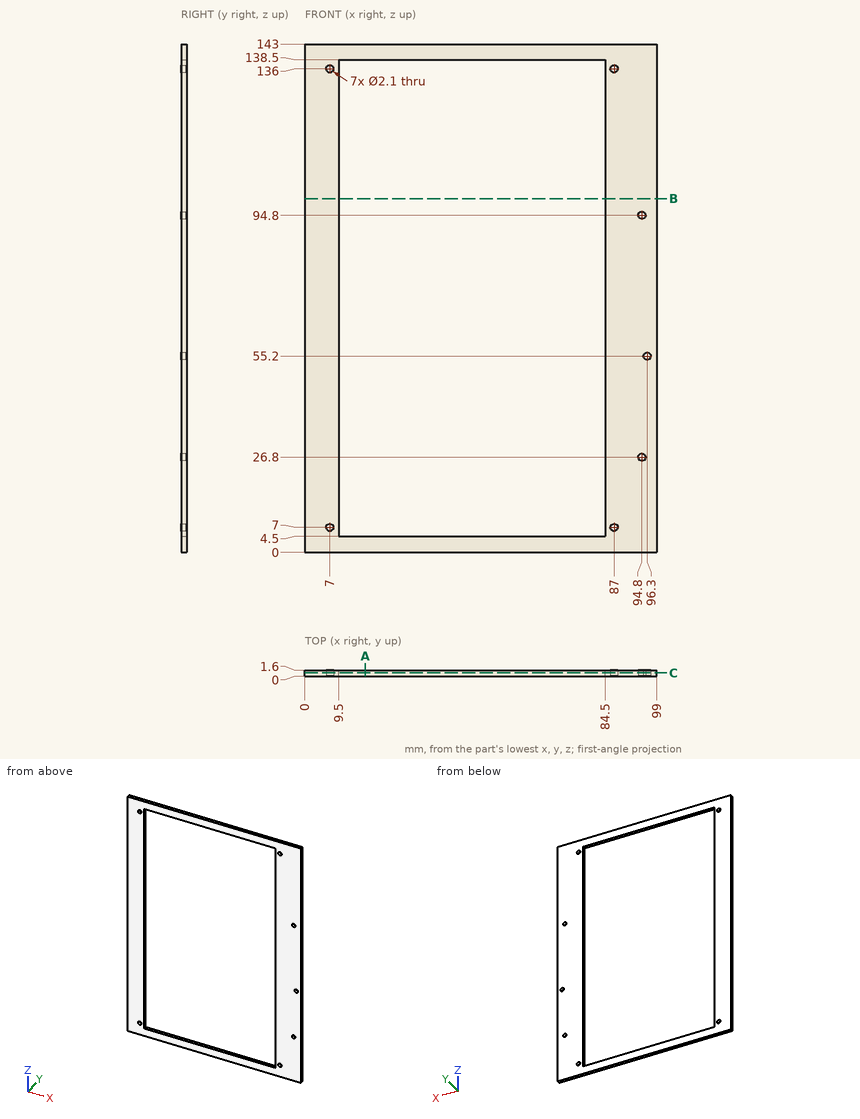
Drawing for the job (mm, zero at the part's lowest x, y, z). Coordinates: 2 decimals unless noted, no trailing zeros. Loops run counter-clockwise (first coordinate to the right, second up) from the corner with the lowest first, then second, coordinate; pieces in that order, holes last. Notation, with made-up numbers: (-39.5, -40) - (-13.5, -40) arc R31 cw to (-13.5, -3) - close; hole circle Ø8 at (-11, 20.25). An arc over 180 degrees is marked (long way). Use CSV: the item, a comma, the result in double quotes. Start each with the question number.
Q1. Drop a flat-ended pin along its axis: P1, Ø2.5, axis at x = 87, z = 7, coming from the +Y side. Give the stop position or say it passes through.
Q2. Cut at B-B, the plane z = 99.5. List the corners of the cut face in (x, y).
Q3. Cut at A-A, the plane x = 17. List the corners of the cut face in (y, z), then the cut area to 3 significant figures.
Q4. Cut at C-C, the plane y = 0.9. State how many separate pieces and enclosed holes the cut face has, then the cut area to 3 significant figures.
Q5. Probe probe 1 along X at (y, z) = (0.85, 136); probe 2 along Z at (x, y) = (87, 1.25); probe 3 along Z at (x, y) = (94.8, 0.5). List the from-to ranges inside material, lowest first. Write a range as from..to.
Here are the results:
1,P1,"y = 1.6"
2,outline,"(0, 0) - (9.5, 0) - (9.5, 1.6) - (0, 1.6) - close; (84.5, 0) - (99, 0) - (99, 1.6) - (84.5, 1.6) - close"
3,outline,"(0, 0) - (1.6, 0) - (1.6, 4.5) - (0, 4.5) - close; (0, 138.5) - (1.6, 138.5) - (1.6, 143) - (0, 143) - close"
3,area,"14.4 mm2"
4,separate pieces,"1"
4,enclosed holes,"8"
4,area,"4,080 mm2"
5,probe 1,"0..5.95, 8.05..9.5, 84.5..85.95, 88.05..99"
5,probe 2,"0..5.95, 8.05..134.95, 137.05..143"
5,probe 3,"0..25.75, 27.85..93.75, 95.85..143"
